The model under review builds one solid part; all positions refer to its coordinate system, in mm. A direction names the side the tool comes from. Round coordinates to 2 decimals unless told otherwise and drop trailing zeros. Order: outer loops, then holes, each group sorted by start corner. A loop starts at its lowest first (then second) coordinate and runs counter-clockwise, first axis right, second up. Notation, with made-up numbers: M 26,65.25 L 65,65.25 A20 cw 65,81.25 Z; hole C -39.5,70.5 d3. An arc over 180 degrees is marked long. Answer as a JSON object with one key per item and string values. Group by question number.
1) Insertion check: pin 1 Ø10.5 at (x, y) = (26.5, 10) entering from +Z; pin 2 Ø1.5 at (x, y) = (12.5, 33) entering from -Z; pin 3 Ø1.1 at (x, z) = (49.5, 29.5) entering from +Y; pin 4 Ø2 at (x, y) = (22, 13) entering from -Z. Each pin has a flat end and moves straight along its axis. Give the tip position at first contact, or say it passes through.
2) Consider section B-B, the plane z = 15. Write out the cut boundary in (x, y), then the cut area to 3 significant figures.
3) For faces 1 (the flat face through (0.8, 13.3, 3.3)), 2 (the flat face through (14, 25, 19)), 3 (the flat face through (13, 49, 24)), list the 3-axis set-ups (+Z, -Z, +X, -X, +Y, -Y) from which the entire face can be reached by the end or side of a thin tool; tool diameter is ignored.
4) To check wall thickness, follow line 1 (X direction, y = 27, z = 14); line 2 (Z direction, x = 43, y = 10). State the ranges of each line that lie inside material, in increasing order.
5) Consider section D-D, the plane x = 40.5. Write out the cut boundary in (y, z), then the cut area to 3 significant figures.
6) Consider section A-A, the plane x = 26.5. Write out the cut boundary in (y, z), then the cut area to 4 significant figures.
7) Consider section C-C, the plane y = 10. Write out the cut boundary in (x, z).
8) The part is to be moulded in two halves that separate along X. For faces 4 (the flat face through (1, 49, 24)), 5 (the flat face through (6.9, 0.8, 24.3)), 6 (the flat face through (49, 1, 1)), 7 (the flat face through (25, 36, 5)), say which applies: +X half, -X half, draft (parallel to the pull), parting line (faces both ways), or undercut.
```python
from build123d import *

# Parameters (mm, degrees)
SKETCH1_W                = 50
SKETCH1_H                = 50
BOSS_EXTRUDE1_DEPTH      = 25
CUT_EXTRUDE1_DEPTH       = 76
CUT_EXTRUDE2_DEPTH       = 76
CUT_EXTRUDE3_DEPTH       = 76
CHAMFER1_SIZE            = 1.5
BOSS_EXTRUDE2_DEPTH      = 7
BOSS_EXTRUDE2_DEPTH_BACK = 10
SKETCH5_W                = 1
SKETCH5_H                = 7
SKETCH6_W                = 1.8
SKETCH6_H                = 1.8
CUT_EXTRUDE5_DEPTH       = 78.614431648


with BuildPart() as part:
    # Sketch1 → Boss-Extrude1 (new body)
    with BuildSketch(Plane.XY):
        with Locations((25, 25)):
            Rectangle(SKETCH1_W, SKETCH1_H)
    extrude(amount=BOSS_EXTRUDE1_DEPTH)

    # Sketch2 → Cut-Extrude1 (cut, through all)
    with BuildSketch(Plane.XZ):
        Polygon((29.556349186, 36), (20.443650814, 36), (14, 29.556349186), (14, 20.443650814), (20.443650814, 14), (29.556349186, 14), (36, 20.443650814), (36, 29.556349186), align=None)
    extrude(amount=-CUT_EXTRUDE1_DEPTH, mode=Mode.SUBTRACT)

    # Sketch3 → Cut-Extrude2 (cut, through all)
    with BuildSketch(Plane.ZY):
        Polygon((4.556349186, 14), (11, 20.443650814), (11, 29.556349186), (4.556349186, 36), (-4.556349186, 36), (-11, 29.556349186), (-11, 20.443650814), (-4.556349186, 14), align=None)
    extrude(amount=-CUT_EXTRUDE2_DEPTH, mode=Mode.SUBTRACT)

    # Sketch4 → Cut-Extrude3 (cut, through all)
    with BuildSketch(Plane.XY.offset(25)):
        Polygon((29.556349186, 36), (20.443650814, 36), (14, 29.556349186), (14, 20.443650814), (20.443650814, 14), (29.556349186, 14), (36, 20.443650814), (36, 29.556349186), align=None)
    extrude(amount=-CUT_EXTRUDE3_DEPTH, mode=Mode.SUBTRACT)

    # Chamfer1
    chamfer1_edges = [part.edges().sort_by_distance(p)[0] for p in [
        (50, 25, 25),
        (43, 50, 25),
        (43, 0, 25),
        (7, 50, 25),
        (14, 25, 25),
        (36, 25, 25),
        (36, 50, 22.721825407),
        (14, 50, 22.721825407),
        (36, 0, 22.721825407),
        (14, 0, 22.721825407),
        (17.221825407, 0, 17.221825407),
        (32.778174593, 0, 17.221825407),
        (32.778174593, 50, 17.221825407),
        (17.221825407, 50, 17.221825407),
        (0, 25, 25),
        (25, 50, 0),
        (50, 7, 0),
        (0, 7, 0),
        (50, 43, 0),
        (25, 36, 0),
        (25, 14, 0),
        (25, 0, 0),
        (0, 43, 0),
        (50, 14, 2.278174593),
        (50, 36, 2.278174593),
        (50, 32.778174593, 7.778174593),
        (50, 17.221825407, 7.778174593),
        (0, 14, 2.278174593),
        (0, 17.221825407, 7.778174593),
        (0, 32.778174593, 7.778174593),
        (0, 36, 2.278174593),
        (7, 0, 25),
        (0, 50, 12.5),
        (50, 50, 12.5),
        (50, 0, 12.5),
        (0, 0, 12.5),
    ]]
    chamfer(chamfer1_edges, length=CHAMFER1_SIZE)

    # Sketch5 → Boss-Extrude2 (add, two sides: drawn at the far end of the back side and taken through both)
    with BuildSketch(Plane.XY.offset(25).offset(-BOSS_EXTRUDE2_DEPTH_BACK)):
        with Locations((49.5, 25)):
            Rectangle(SKETCH5_W, SKETCH5_H)
    extrude(amount=BOSS_EXTRUDE2_DEPTH + BOSS_EXTRUDE2_DEPTH_BACK)

    # Sketch6 → Cut-Extrude5 (cut, through all)
    with BuildSketch(Plane(origin=(50, 0, 0), x_dir=(0, 0, -1), z_dir=(1, 0, 0))):
        with Locations((-28.6, 25)):
            Rectangle(SKETCH6_W, SKETCH6_H)
    extrude(amount=-CUT_EXTRUDE5_DEPTH, mode=Mode.SUBTRACT)


solid = part.part
```
Results list:
{
 "1": {"pin 1": "z = 16.19", "pin 2": "z = 6.81", "pin 3": "y = 28.5", "pin 4": "z = 0"},
 "2": {"outline": "M 0,1.5 L 1.5,0 L 17.32,0 L 19.44,1.5 L 19.44,15 L 14,20.44 L 14,29.56 L 19.44,35 L 19.44,48.5 L 17.32,50 L 1.5,50 L 0,48.5 Z; M 30.56,1.5 L 32.68,0 L 48.5,0 L 50,1.5 L 50,48.5 L 48.5,50 L 32.68,50 L 30.56,48.5 L 30.56,35 L 36,29.56 L 36,20.44 L 30.56,15 Z", "area": "1,780 mm^2"},
 "3": {"face 1": "-Z, -X", "face 2": "+Z", "face 3": "+Z, +Y"},
 "4": {"line 1": "0 to 14, 36 to 50", "line 2": "0 to 25"},
 "5": {"outline": "M 0,1.5 L 1.5,0 L 12.5,0 L 14,1.5 L 14,4.56 L 20.44,11 L 29.56,11 L 36,4.56 L 36,1.5 L 37.5,0 L 48.5,0 L 50,1.5 L 50,23.5 L 48.5,25 L 1.5,25 L 0,23.5 Z", "area": "1,040 mm^2"},
 "6": {"outline": "M 0,1.5 L 1.5,0 L 12.5,0 L 14,1.5 L 14,14 L 0,14 Z; M 36,1.5 L 37.5,0 L 48.5,0 L 50,1.5 L 50,14 L 36,14 Z", "area": "387.5 mm^2"},
 "7": {"outline": "M 0,1.5 L 1.5,0 L 48.5,0 L 50,1.5 L 50,23.5 L 48.5,25 L 37.5,25 L 36,23.5 L 36,20.44 L 29.56,14 L 20.44,14 L 14,20.44 L 14,23.5 L 12.5,25 L 1.5,25 L 0,23.5 Z"},
 "8": {"face 4": "-X half", "face 5": "draft", "face 6": "+X half", "face 7": "undercut"}
}
